Study the drawing (mm; zero at the part's minimum x, y, z) and answer. A direction names the side the tool comes from. Give positions to 0.01 mm unless a question says otherwise; leave off trailing zeros. Write each loop counter-clockwise with the first axis right and the second up, starting at its lowest first coordinate (ties: lowest second). Pieces come first, ordered by that corner, then holes. Notation, with made-up numbers: (-16.5, 32.5) - (12.5, 32.5) arc R16 ccw to (12.5, 49.5) - close; hole circle Ø1 at (39.5, -39.75). An arc over 180 degrees is marked (long way). Return JSON: item names as keys, results as strings.
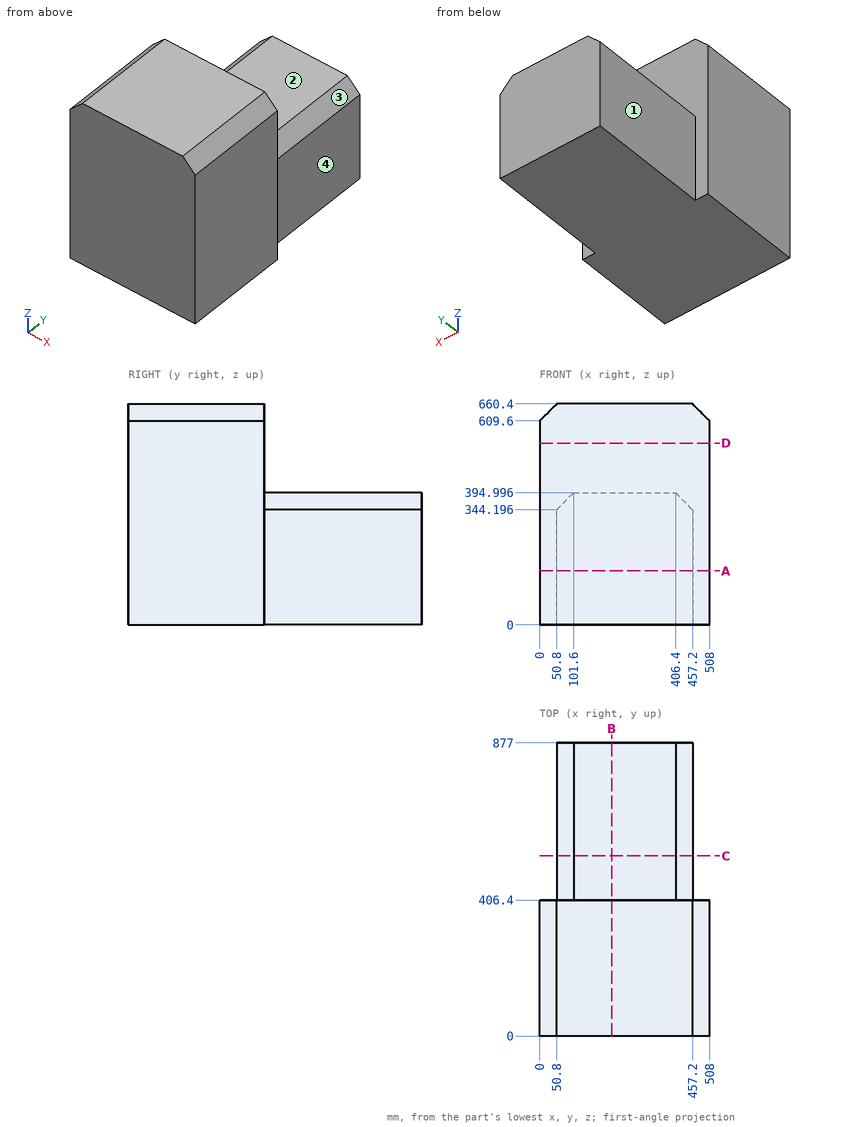
Item 1: Consider L1, parallel to Z at x = 374, y = 817; L2, parallel to Y at x = 77, z = 584; L3, parallel to X at y = 428, z = 118. Determine where each line is inside the solid, lowest interval first.
Answer below:
{"L1": "z = 0 to 395", "L2": "y = 0 to 406.4", "L3": "x = 50.8 to 457.2"}
Item 2: For the marked faces 1, 2, 3 and 4, determine the directions among +Z, -Z, +X, -X, +Y, -Y from which every point of the face is accessible in a straight line to the end or side of a thin tool.
Answer below:
{"face 1": "+Z, -Z, -X, +Y", "face 2": "+Z, +X, -X, +Y", "face 3": "+Z, +X, +Y", "face 4": "+Z, -Z, +X, +Y"}
Item 3: A cutting plane is placed at B-B on x = 215. Determine the outline of the cut face in (y, z).
Answer below:
{"outline": "(0, 0) - (877, 0) - (877, 395) - (406.4, 395) - (406.4, 660.4) - (0, 660.4) - close"}
Item 4: Flat-ended cylindrical pins translate along their axes: P1, Ø10, axis at x = 90, y = 560, coming from the +Z side; P2, Ø4, axis at y = 765.5, z = 321.5, coming from the +X side; P3, Ø1, axis at x = 183.5, y = 441, coming from the +Z side. Find the tip coordinate at first contact, or state that the pin passes through.
Answer below:
{"P1": "stops at z = 388.4", "P2": "stops at x = 457.2", "P3": "stops at z = 395"}
Item 5: A cutting plane is placed at D-D on z = 543. Determine the outline of the cut face in (x, y).
Answer below:
{"outline": "(0, 0) - (508, 0) - (508, 406.4) - (0, 406.4) - close"}
Item 6: A cutting plane is placed at A-A on z = 161.5. Determine the outline of the cut face in (x, y).
Answer below:
{"outline": "(0, 0) - (508, 0) - (508, 406.4) - (457.2, 406.4) - (457.2, 877) - (50.8, 877) - (50.8, 406.4) - (0, 406.4) - close"}
Item 7: A cutting plane is placed at C-C on y = 538.5. Determine the outline of the cut face in (x, z), then the cut area to 3 significant figures.
Answer below:
{"outline": "(50.8, 0) - (457.2, 0) - (457.2, 344.2) - (406.4, 395) - (101.6, 395) - (50.8, 344.2) - close", "area": "158,000 mm²"}
